Could you check a few things on this model? Use its own coordinates, in mm. Face numbers are marked on the shaded views. A direction names the side the tool comes from. Give positions to 0.01 mm unless a question says otherwise; leave off trailing zeros. Order: outer loops, then holes, each group sorted by start corner. A loop starts at its lowest first (then second) coordinate and runs counter-clockwise, first axis right, second up.
(1) Imagine slicing it at B-B, the plane y = 40. Write out the boundary of the cut face in (x, z).
(2) On a 3-axis mill with a long thin cutter (end or side, diameter ignored), from which of +Z, -Z, +X, -X, +Y, -Y can I reach the whole of each face in a straight line? I mean the marked faces 4, 5 and 6. Say none if no direction works.
(3) If we mould it in two halves opening along X, with no side actions, what happens to the marked faces 1, 2 and 3? For each: released by +X, released by -X, zero draft, split by the parting line, or undercut.
(4) If I drill on probe 1 along Y at (x, z) = (90, -4); probe 2 along X at (y, z) = (-4, 10.75); probe 3 along X at (y, z) = (5, -1.25), over which ranges is the centre line in solid material (lowest first)?
(5) Imagine slicing it at C-C, the plane z = 12. Write out the boundary of the cut face in (x, y), then the cut area to 3 significant figures.
(6) Imagine slicing it at D-D, the plane y = -26.5. Write out the boundary of the cut face in (x, z).
(7) Imagine slicing it at A-A, the plane x = 90. Write out the boundary of the cut face in (y, z), then the cut area to 3 significant figures.
(8) Will these pins go through, and if not, where does the flat tip stop? pin 1 (6.5 mm diameter, centred on x = 90, y = 10, fed in from +Z); pin 2 (15 mm diameter, centred on x = -6.5, y = -34.5, fed in from +Z).
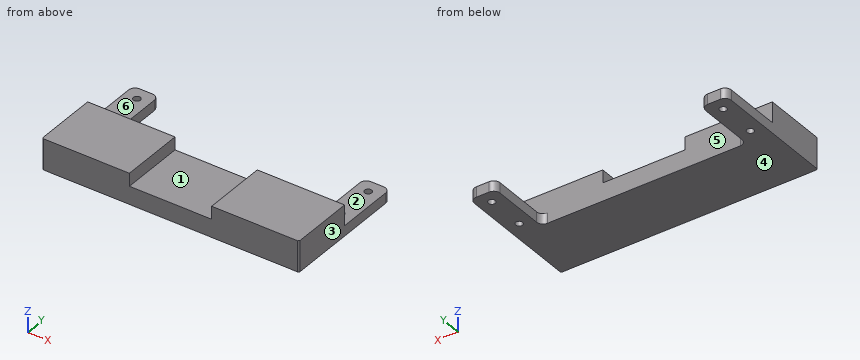
from build123d import *

# Parameters (mm, degrees)
BOSS_EXTRUDE1_DEPTH  = 50
SKETCH2_W            = 20
SKETCH2_H            = 8
BOSS_EXTRUDE2_DEPTH  = 50
M5_CLEARANCE_HOLE1_D = 5.5
FILLET1_R            = 5
CHAMFER1_SIZE        = 1


with BuildPart() as part:
    # Sketch1 → Boss-Extrude1 (new body)
    with BuildSketch(Plane(origin=(0, 0, 0), x_dir=(1, 0, 0), z_dir=(0, 1, 0))):
        Polygon((-100, 8), (100, 8), (100, -16), (32, -16), (32, -6), (-32, -6), (-32, -16), (-100, -16), align=None)
    extrude(amount=-BOSS_EXTRUDE1_DEPTH)

    # Sketch2 → Boss-Extrude2 (add)
    with BuildSketch(Plane(origin=(0, 0, 0), x_dir=(1, 0, 0), z_dir=(0, 1, 0))):
        with Locations((-90, 4)):
            Rectangle(SKETCH2_W, SKETCH2_H)
        with Locations((90, 4)):
            Rectangle(SKETCH2_W, SKETCH2_H)
    extrude(amount=BOSS_EXTRUDE2_DEPTH)

    # M5 Clearance Hole1 (through all)
    with Locations(Plane(origin=(0, 0, -8), x_dir=(-1, 0, 0), z_dir=(0, 0, -1))):
        with Locations((-90, 40), (90, 10), (-90, 10), (90, 40)):
            Hole(M5_CLEARANCE_HOLE1_D / 2)

    # Fillet1
    fillet1_edges = [part.edges().sort_by_distance(p)[0] for p in [
        (-80, 0, -4),
        (-100, 50, -4),
        (-80, 50, -4),
        (80, 0, -4),
        (100, 50, -4),
        (80, 50, -4),
    ]]
    fillet(fillet1_edges, radius=FILLET1_R)

    # Chamfer1
    chamfer1_edges = [part.edges().sort_by_distance(p)[0] for p in [
        (100, -50, 4),
        (-100, -50, 4),
    ]]
    chamfer(chamfer1_edges, length=CHAMFER1_SIZE)


solid = part.part
Answer block:
1. outline: (-100, -8) - (-92.75, -8) - (-92.75, 0) - (-100, 0) - close; (-87.25, -8) - (-80, -8) - (-80, 0) - (-87.25, 0) - close; (80, -8) - (87.25, -8) - (87.25, 0) - (80, 0) - close; (92.75, -8) - (100, -8) - (100, 0) - (92.75, 0) - close
2. face 4: -Z, +X, -X, +Y, -Y
2. face 5: +Z, +Y
2. face 6: +Z, +X, -X, +Y
3. face 1: undercut
3. face 2: zero draft
3. face 3: released by +X
4. probe 1: y = -50 to 7.25, 12.75 to 37.25, 42.75 to 50
4. probe 2: x = -100 to -32, 32 to 100
4. probe 3: x = -100 to -80, 80 to 100
5. outline: (-100, -49) - (-99, -50) - (-32, -50) - (-32, 0) - (-100, 0) - close; (32, -50) - (99, -50) - (100, -49) - (100, 0) - (32, 0) - close
5. area: 6,800 mm2
6. outline: (-100, -8) - (100, -8) - (100, 16) - (32, 16) - (32, 6) - (-32, 6) - (-32, 16) - (-100, 16) - close
7. outline: (-50, -8) - (7.25, -8) - (7.25, 0) - (0, 0) - (0, 16) - (-50, 16) - close; (12.75, -8) - (37.25, -8) - (37.25, 0) - (12.75, 0) - close; (42.75, -8) - (50, -8) - (50, 0) - (42.75, 0) - close
7. area: 1,510 mm2
8. pin 1: stops at z = 0
8. pin 2: stops at z = 6
